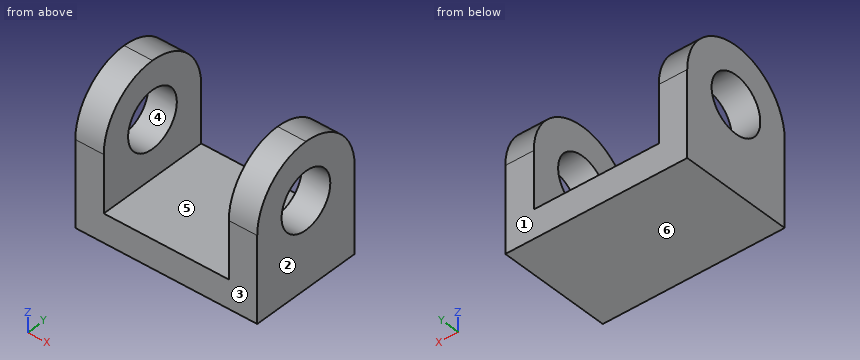
```python
from build123d import *

# Parameters (mm, degrees)
SKETCH1_W           = 40.64
SKETCH1_H           = 25.4
BOSS_EXTRUDE1_DEPTH = 31.75
SKETCH3_W           = 27.94
SKETCH3_H           = 25.4
CUT_EXTRUDE1_DEPTH  = 26.4
SKETCH4_R           = 6.35
CUT_EXTRUDE2_DEPTH  = 41.64
CUT_EXTRUDE3_DEPTH  = 41.64


with BuildPart() as part:
    # Sketch1 → Boss-Extrude1 (new body)
    with BuildSketch(Plane.XY):
        Rectangle(SKETCH1_W, SKETCH1_H)
    extrude(amount=BOSS_EXTRUDE1_DEPTH)

    # Sketch3 → Cut-Extrude1 (cut, through all)
    with BuildSketch(Plane(origin=(0, 12.7, 0), x_dir=(1, 0, 0), z_dir=(0, 1, 0))):
        with Locations((0, -19.05)):
            Rectangle(SKETCH3_W, SKETCH3_H)
    extrude(amount=-CUT_EXTRUDE1_DEPTH, mode=Mode.SUBTRACT)

    # Sketch4 → Cut-Extrude2 (cut, through all)
    with BuildSketch(Plane(origin=(20.32, 0, 0), x_dir=(0, 0, -1), z_dir=(1, 0, 0))):
        with Locations(Location((-19.05, 0, 0), (0, 0, 90))):  # turned: the seam where the file's is
            Circle(SKETCH4_R)
    extrude(amount=-CUT_EXTRUDE2_DEPTH, mode=Mode.SUBTRACT)

    # Sketch5 → Cut-Extrude3 (cut, through all)
    with BuildSketch(Plane(origin=(20.32, 0, 0), x_dir=(0, 0, -1), z_dir=(1, 0, 0))):
        with BuildLine():
            Line((-31.75, 12.7), (-19.05, 12.7))
            ThreePointArc((-19.05, 12.7), (-28.030256121, 8.980256121), (-31.75, 0))
            Line((-31.75, 0), (-31.75, 12.7))
        make_face()
    cut_extrude3 = extrude(amount=-CUT_EXTRUDE3_DEPTH, mode=Mode.SUBTRACT)

    # Mirror1: Cut-Extrude3 across plane
    add(cut_extrude3.mirror(Plane.ZX), mode=Mode.SUBTRACT)


solid = part.part
```
Build history of the part. All positions in model axes, mm. Face numbers are marked on the shaded views. A direction names the side the tool comes from. Round coordinates to 2 decimals unless told otherwise and drop trailing zeros. Write each loop counter-clockwise with the first axis right and the second up, starting at its lowest first coordinate (ties: lowest second). Pieces come first, ordered by that corner, then holes.
1) Pin check, flat tips, straight feed: pin 1 (3 mm diameter, centred on x = -8, y = 0, fed in from +Z); pin 2 (10 mm diameter, centred on x = -7, z = 16, fed in from +Y); pin 3 (10 mm diameter, centred on x = -9.5, z = 23.5, fed in from +Y); pin 4 (1.5 mm diameter, centred on x = -16, z = 27, fed in from +Y). Stop position of each tip, or through.
2) Band-saw the part on A-A, the plane z = 10. List the corners of the cut face in (x, y).
3) Band-saw the part on B-B, the plane y = -4. List the corners of the cut face in (x, z).
4) 3-axis set-ups, long thin cutter, end or side, ignore diameter. For the marked faces 5 and 6: which of +Z, -Z, +X, -X, +Y, -Y reach the whole face in a straight line?
5) Drill centre lines: probe 1 along X at (y, z) = (8.75, 22); probe 2 along Y at (x, z) = (16, 19); probe 3 along Z at (x, y) = (-19, 0). Where is each one in solid material? Low to high.
6) Band-saw the part on D-D, the plane y = 10.5. List the corners of the cut face in (x, z), and give its area (3 significant figures).
7) Band-saw the part on C-C, the plane x = -14.5. List the corners of the cut face in (y, z), and give its area (3 significant figures).
8) Mould opens along Y. For the marked faces 1, 2, 3 and 4 say: +Y half, -Y half, draft (parallel to the pull), parting line (faces both ways), or undercut.
Ans:
1. pin 1: stops at z = 6.35
1. pin 2: passes through
1. pin 3: stops at y = 12.51
1. pin 4: stops at y = 10.46
2. outline: (-20.32, -12.7) - (-13.97, -12.7) - (-13.97, 12.7) - (-20.32, 12.7) - close; (13.97, -12.7) - (20.32, -12.7) - (20.32, 12.7) - (13.97, 12.7) - close
3. outline: (-20.32, 0) - (20.32, 0) - (20.32, 14.12) - (13.97, 14.12) - (13.97, 6.35) - (-13.97, 6.35) - (-13.97, 14.12) - (-20.32, 14.12) - close; (-20.32, 23.98) - (-13.97, 23.98) - (-13.97, 31.1) - (-20.32, 31.1) - close; (13.97, 23.98) - (20.32, 23.98) - (20.32, 31.1) - (13.97, 31.1) - close
4. face 5: +Z, +Y, -Y
4. face 6: -Z, +X, -X, +Y, -Y
5. probe 1: x = -20.32 to -13.97, 13.97 to 20.32
5. probe 2: y = -12.7 to -6.35, 6.35 to 12.7
5. probe 3: z = 0 to 12.7, 25.4 to 31.75
6. outline: (-20.32, 0) - (20.32, 0) - (20.32, 26.19) - (13.97, 26.19) - (13.97, 6.35) - (-13.97, 6.35) - (-13.97, 26.19) - (-20.32, 26.19) - close
6. area: 510 mm2
7. outline: (-12.7, 0) - (12.7, 0) - (12.7, 19.05) arc R12.7 ccw to (-12.7, 19.05) - close; hole circle Ø12.7 at (0, 19.05)
7. area: 611 mm2
8. face 1: +Y half
8. face 2: draft
8. face 3: -Y half
8. face 4: undercut
